Verification items for the finished model (mm, model axes). A direction names the side the tool comes from. Give positions to 0.01 mm unless a question says otherwise; leave off trailing zeros. Order: outer loops, then holes, each group sorted by start corner. A loop starts at its lowest first (then second) coordinate and runs counter-clockwise, first axis right, second up.
(1) Mould release check, pull along Z, two halves, no side actions. Record for faces 5 (the face through (-43, 2, -21.897)), 6 (the face through (-26.148, 1.933, -20.883)), 7 (the face through (-42, 3, -12)): pulls with the +Z half, pulls with the -Z half, needs draft (parallel to the pull), parting line crosses it, or undercut.
(2) Sectioned sample at A-A on z = -11.5. Record the cut outline in (x, y).
(3) Sectioned sample at B-B on x = -23. Record the cut outline in (y, z).
(4) Access from +Z, -Z, +X, -X, +Y, -Y to the whole of each face (thin tool, end or side, straight path). Record for faces 1 (the face through (-8.947, 2, -12)), 2 (the face through (-44.06, 2.23, -20.88)), 3 (the face through (-21.675, 2, -11)), 4 (the face through (-30, 2, -18.897)).
(5) Gauge pin test, flat ends, axial feed: pin 1 (2.5 mm diameter, centred on x = -25, y = 3, fed in from +Z); pin 2 (1.2 mm diameter, centred on x = -44, y = 2.5, fed in from +Z); pin 3 (0.8 mm diameter, centred on y = 1.5, z = -19.5, fed in from -X). Record the tip position at first contact, or that the pin passes through.
(6) Scan lines: L1, parallel to X at y = 2.5, z = -19; L2, parallel to X at y = 1.75, z = 0; L3, parallel to X at y = 2, z = -13. Record each from-to range of solid material in increasing order.
```python
from build123d import *

# Parameters (mm, degrees)
SKETCH1_W            = 55
SKETCH1_H            = 30
BOSS_EXTRUDE1_DEPTH  = 1
SKETCH2_W            = 19.491695939
SKETCH2_H            = 7.592367472
BOSS_EXTRUDE2_DEPTH  = 1
SKETCH3_W            = 17.868683869
SKETCH3_H            = 5.806480893
BOSS_EXTRUDE3_DEPTH  = 5
SKETCH4_R            = 1.387992379
SKETCH4_R_2          = 1.271029941
SKETCH4_R_3          = 1.252160081
SKETCH4_R_4          = 1.29898612
SKETCH4_R_5          = 1.250669325
CUT_EXTRUDE1_DEPTH   = 1
SKETCH5_W            = 10.590314041
SKETCH5_H            = 7.273255242
BOSS_EXTRUDE4_DEPTH  = 1
SKETCH6_W            = 9.57185552
SKETCH6_H            = 5.896073661
BOSS_EXTRUDE5_DEPTH  = 5
SKETCH7_R            = 1.704864166
SKETCH7_R_2          = 1.652773159
CUT_EXTRUDE2_DEPTH   = 1
SKETCH8_W            = 4.39691748
SKETCH8_H            = 1.56078367
SKETCH8_H_2          = 1.965861173
SKETCH8_H_3          = 1.923435972
BOSS_EXTRUDE6_DEPTH  = 3
SKETCH9_W            = 3.511257789
SKETCH9_H            = 7.74384092
SKETCH9_W_2          = 2.828211164
SKETCH9_W_3          = 3.357629357
SKETCH9_H_2          = 9.12002374
SKETCH9_W_4          = 3.515822041
BOSS_EXTRUDE7_DEPTH  = 2
SKETCH11_W           = 9.526847307
SKETCH11_H           = 2.580834009
BOSS_EXTRUDE9_DEPTH  = 1
SKETCH12_W           = 10.214883885
SKETCH12_H           = 2.399198827
BOSS_EXTRUDE10_DEPTH = 1
SKETCH13_W           = 9.211002793
SKETCH13_H           = 2.314821269
BOSS_EXTRUDE11_DEPTH = 1
SKETCH14_W           = 8.269131958
SKETCH14_H           = 2.253083688
BOSS_EXTRUDE12_DEPTH = 1
SKETCH15_R           = 2.31957405
SKETCH15_R_2         = 2.335420551
SKETCH15_R_3         = 2.850653073
SKETCH15_R_4         = 3.324876744
BOSS_EXTRUDE13_DEPTH = 5
SKETCH16_R           = 1.17518149
SKETCH16_R_2         = 1.252285298
SKETCH16_R_3         = 1.321478457
SKETCH16_R_4         = 1.276209415
CUT_EXTRUDE3_DEPTH   = 5
SKETCH17_W           = 3.572088618
SKETCH17_H           = 5.777043793
SKETCH17_W_2         = 3.071926892
SKETCH17_H_2         = 6.434501435
CUT_EXTRUDE4_DEPTH   = 5
SKETCH18_W           = 6.981016606
SKETCH18_H           = 6.578879703
SKETCH18_W_2         = 3.086522126
SKETCH18_H_2         = 3.227214814
SKETCH18_W_3         = 3.221722133
SKETCH18_H_3         = 3.240258565
SKETCH18_W_4         = 3.482439067
SKETCH18_H_4         = 3.404908775
BOSS_EXTRUDE14_DEPTH = 2
SKETCH19_R           = 0.719775063
SKETCH19_R_2         = 0.76029107
SKETCH19_R_3         = 0.758288133
SKETCH19_R_4         = 0.716718546
SKETCH19_R_5         = 0.645890237
SKETCH19_R_6         = 0.78925264
SKETCH19_R_7         = 0.788868737
SKETCH19_R_8         = 0.878549595
SKETCH19_R_9         = 0.90829019
SKETCH19_R_10        = 0.920218082
SKETCH19_R_11        = 0.847809832
SKETCH19_R_12        = 0.813287674
BOSS_EXTRUDE15_DEPTH = 2
SKETCH20_W           = 2.420557599
SKETCH20_H           = 3.478717889
BOSS_EXTRUDE17_DEPTH = 4
SKETCH22_W           = 1.956579844
SKETCH22_H           = 2.647802663
BOSS_EXTRUDE19_DEPTH = 4
SKETCH23_R           = 0.740483371
BOSS_EXTRUDE20_DEPTH = 3


with BuildPart() as part:
    # Sketch1 → Boss-Extrude1 (new body)
    with BuildSketch(Plane(origin=(0, 0, 0), x_dir=(1, 0, 0), z_dir=(0, 1, 0))):
        with Locations((-21.264064322, 3.89729895)):
            Rectangle(SKETCH1_W, SKETCH1_H)
    extrude(amount=BOSS_EXTRUDE1_DEPTH)

    # Sketch2 → Boss-Extrude2 (add)
    with BuildSketch(Plane(origin=(0, 1, 0), x_dir=(1, 0, 0), z_dir=(0, 1, 0))):
        with Locations((-5.49817758, -4.994329297)):
            Rectangle(SKETCH2_W, SKETCH2_H)
    extrude(amount=BOSS_EXTRUDE2_DEPTH)

    # Sketch3 → Boss-Extrude3 (add)
    with BuildSketch(Plane(origin=(0, 2, 0), x_dir=(1, 0, 0), z_dir=(0, 1, 0))):
        with Locations((-5.399712824, -5.130077774)):
            Rectangle(SKETCH3_W, SKETCH3_H)
    extrude(amount=BOSS_EXTRUDE3_DEPTH)

    # Sketch4 → Cut-Extrude1 (cut)
    with BuildSketch(Plane(origin=(0, 7, 0), x_dir=(1, 0, 0), z_dir=(0, 1, 0))):
        with Locations(Location((-12.18713871, -5.16756273, 0), (0, 0, 270))):
            Circle(SKETCH4_R)
        with Locations(Location((-8.689373295, -5.16756273, 0), (0, 0, 270))):
            Circle(SKETCH4_R_2)
        with Locations(Location((-5.533968846, -5.16756273, 0), (0, 0, 270))):
            Circle(SKETCH4_R_3)
        with Locations(Location((-2.349125846, -5.16756273, 0), (0, 0, 270))):
            Circle(SKETCH4_R_4)
        with Locations(Location((0.92403281, -5.16756273, 0), (0, 0, 270))):
            Circle(SKETCH4_R_5)
    extrude(amount=-CUT_EXTRUDE1_DEPTH, mode=Mode.SUBTRACT)

    # Sketch5 → Boss-Extrude4 (add)
    with BuildSketch(Plane(origin=(0, 1, 0), x_dir=(1, 0, 0), z_dir=(0, 1, 0))):
        with Locations((-20.994245653, -4.916719061)):
            Rectangle(SKETCH5_W, SKETCH5_H)
    extrude(amount=BOSS_EXTRUDE4_DEPTH)

    # Sketch6 → Boss-Extrude5 (add)
    with BuildSketch(Plane(origin=(0, 2, 0), x_dir=(1, 0, 0), z_dir=(0, 1, 0))):
        with Locations((-21.014512422, -4.903762727)):
            Rectangle(SKETCH6_W, SKETCH6_H)
    extrude(amount=BOSS_EXTRUDE5_DEPTH)

    # Sketch7 → Cut-Extrude2 (cut)
    with BuildSketch(Plane(origin=(0, 7, 0), x_dir=(1, 0, 0), z_dir=(0, 1, 0))):
        with Locations(Location((-23.578627502, -4.834787204, 0), (0, 0, 270))):
            Circle(SKETCH7_R)
        with Locations(Location((-19.287367013, -4.834787204, 0), (0, 0, 270))):
            Circle(SKETCH7_R_2)
    extrude(amount=-CUT_EXTRUDE2_DEPTH, mode=Mode.SUBTRACT)

    # Sketch8 → Boss-Extrude6 (add)
    with BuildSketch(Plane(origin=(0, 1, 0), x_dir=(1, 0, 0), z_dir=(0, 1, 0))):
        with Locations((-23.873740649, 14.984908312)):
            Rectangle(SKETCH8_W, SKETCH8_H)
        with Locations((-23.873740649, 11.393249572)):
            Rectangle(SKETCH8_W, SKETCH8_H_2)
        with Locations((-23.873740649, 7.106266144)):
            Rectangle(SKETCH8_W, SKETCH8_H_3)
    extrude(amount=BOSS_EXTRUDE6_DEPTH)

    # Sketch9 → Boss-Extrude7 (add)
    with BuildSketch(Plane(origin=(0, 1, 0), x_dir=(1, 0, 0), z_dir=(0, 1, 0))):
        with Locations((-41.824470852, 11.59406106)):
            Rectangle(SKETCH9_W, SKETCH9_H)
        with Locations((-34.376000541, 11.59406106)):
            Rectangle(SKETCH9_W_2, SKETCH9_H)
        with Locations((-10.62597461, 12.28215247)):
            Rectangle(SKETCH9_W_3, SKETCH9_H_2)
        with Locations((-4.140862927, 12.28215247)):
            Rectangle(SKETCH9_W_4, SKETCH9_H_2)
    extrude(amount=BOSS_EXTRUDE7_DEPTH)

    # Sketch11 → Boss-Extrude9 (add)
    with BuildSketch(Plane(origin=(0, 0, -18.89729895), x_dir=(-1, 0, 0), z_dir=(0, 0, -1))):
        with Locations((43.030759371, 2.129646377)):
            Rectangle(SKETCH11_W, SKETCH11_H)
    extrude(amount=BOSS_EXTRUDE9_DEPTH)

    # Sketch12 → Boss-Extrude10 (add)
    with BuildSketch(Plane(origin=(0, 0, -18.89729895), x_dir=(-1, 0, 0), z_dir=(0, 0, -1))):
        with Locations((30.43046596, 2.006084235)):
            Rectangle(SKETCH12_W, SKETCH12_H)
    extrude(amount=BOSS_EXTRUDE10_DEPTH)

    # Sketch13 → Boss-Extrude11 (add)
    with BuildSketch(Plane(origin=(0, 0, -18.89729895), x_dir=(-1, 0, 0), z_dir=(0, 0, -1))):
        with Locations((12.330175076, 2.015979145)):
            Rectangle(SKETCH13_W, SKETCH13_H)
    extrude(amount=BOSS_EXTRUDE11_DEPTH)

    # Sketch14 → Boss-Extrude12 (add)
    with BuildSketch(Plane(origin=(0, 0, -18.89729895), x_dir=(-1, 0, 0), z_dir=(0, 0, -1))):
        with Locations((1.581311109, 1.994768123)):
            Rectangle(SKETCH14_W, SKETCH14_H)
    extrude(amount=BOSS_EXTRUDE12_DEPTH)

    # Sketch15 → Boss-Extrude13 (add)
    with BuildSketch(Plane(origin=(0, 1, 0), x_dir=(1, 0, 0), z_dir=(0, 1, 0))):
        with Locations(Location((-7.252523926, 2.900653957, 0), (0, 0, 270))):
            Circle(SKETCH15_R)
        with Locations(Location((-1.058148133, 2.900653957, 0), (0, 0, 270))):
            Circle(SKETCH15_R_2)
        with Locations(Location((-33.782017374, -5.710655696, 0), (0, 0, 270))):
            Circle(SKETCH15_R_3)
        with Locations(Location((-43.660307349, -5.710655696, 0), (0, 0, 270))):
            Circle(SKETCH15_R_4)
    extrude(amount=BOSS_EXTRUDE13_DEPTH)

    # Sketch16 → Cut-Extrude3 (cut)
    with BuildSketch(Plane(origin=(0, 1, 0), x_dir=(1, 0, 0), z_dir=(0, 1, 0))):
        with Locations((-51.576522497, 22.016727671)):
            Circle(SKETCH16_R)
        with Locations((-51.576522497, -8.848199257)):
            Circle(SKETCH16_R_2)
        with Locations((4.236348916, 22.016727671)):
            Circle(SKETCH16_R_3)
        with Locations(Location((4.71641652, -9.248882224, 0), (0, 0, 270))):
            Circle(SKETCH16_R_4)
    extrude(amount=-CUT_EXTRUDE3_DEPTH, mode=Mode.SUBTRACT)

    # Sketch17 → Cut-Extrude4 (cut)
    with BuildSketch(Plane(origin=(0, 1, 0), x_dir=(1, 0, 0), z_dir=(0, 1, 0))):
        with Locations((-52.185475992, 15.830959354)):
            Rectangle(SKETCH17_W, SKETCH17_H)
        with Locations((5.809579957, 14.174599881)):
            Rectangle(SKETCH17_W_2, SKETCH17_H_2)
    extrude(amount=-CUT_EXTRUDE4_DEPTH, mode=Mode.SUBTRACT)

    # Sketch18 → Boss-Extrude14 (add)
    with BuildSketch(Plane(origin=(0, 1, 0), x_dir=(1, 0, 0), z_dir=(0, 1, 0))):
        with Locations((-33.773534226, 1.886893529)):
            Rectangle(SKETCH18_W, SKETCH18_H)
        with Locations((-46.681665239, 4.480707082)):
            Rectangle(SKETCH18_W_2, SKETCH18_H_2)
        with Locations((-41.483525563, 0.631278088)):
            Rectangle(SKETCH18_W_3, SKETCH18_H_3)
        with Locations((-17.396903315, 16.139817099)):
            Rectangle(SKETCH18_W_4, SKETCH18_H_4)
    extrude(amount=BOSS_EXTRUDE14_DEPTH)

    # Sketch19 → Boss-Extrude15 (add)
    with BuildSketch(Plane(origin=(0, 0, -19.89729895), x_dir=(-1, 0, 0), z_dir=(0, 0, -1))):
        with Locations((-1.366958386, 1.973684487)):
            Circle(SKETCH19_R)
        with Locations((1.106822062, 1.973684487)):
            Circle(SKETCH19_R_2)
        with Locations((3.600495928, 1.795519179)):
            Circle(SKETCH19_R_3)
        with Locations((9.279826449, 1.973684487)):
            Circle(SKETCH19_R_4)
        with Locations((11.619345424, 1.795519179)):
            Circle(SKETCH19_R_5)
        with Locations((14.413821044, 1.795519179)):
            Circle(SKETCH19_R_6)
        with Locations((26.935713498, 1.898398295)):
            Circle(SKETCH19_R_7)
        with Locations((29.585968295, 1.898398295)):
            Circle(SKETCH19_R_8)
        with Locations((32.353085369, 1.898398295)):
            Circle(SKETCH19_R_9)
        with Locations((40.159649939, 1.898398295)):
            Circle(SKETCH19_R_10)
        with Locations((43.252965878, 1.973684487)):
            Circle(SKETCH19_R_11)
        with Locations((45.626690014, 1.973684487)):
            Circle(SKETCH19_R_12)
    extrude(amount=BOSS_EXTRUDE15_DEPTH)

    # Sketch20 → Boss-Extrude17 (add)
    with BuildSketch(Plane(origin=(0, 1, 0), x_dir=(1, 0, 0), z_dir=(0, 1, 0))):
        with Locations((-45.209433873, -0.39597322)):
            Rectangle(SKETCH20_W, SKETCH20_H)
    extrude(amount=BOSS_EXTRUDE17_DEPTH)

    # Sketch22 → Boss-Extrude19 (add)
    with BuildSketch(Plane(origin=(0, 1, 0), x_dir=(1, 0, 0), z_dir=(0, 1, 0))):
        with Locations((3.480988959, 4.090806431)):
            Rectangle(SKETCH22_W, SKETCH22_H)
    extrude(amount=BOSS_EXTRUDE19_DEPTH)

    # Sketch23 → Boss-Extrude20 (add)
    with BuildSketch(Plane(origin=(4.459278881, 0, 0), x_dir=(0, 0, -1), z_dir=(1, 0, 0))):
        with Locations(Location((4.071876489, 3.501691713, 0), (0, 0, 180))):
            Circle(SKETCH23_R)
    extrude(amount=BOSS_EXTRUDE20_DEPTH)


solid = part.part
```
Ans:
1. face 5: pulls with the -Z half
1. face 6: needs draft
1. face 7: undercut
2. outline: (-48.76, 0) - (4.27, 0) - (4.27, 1) - (-2.38, 1) - (-2.38, 3) - (-5.9, 3) - (-5.9, 1) - (-8.95, 1) - (-8.95, 3) - (-12.3, 3) - (-12.3, 1) - (-21.68, 1) - (-21.68, 4) - (-26.07, 4) - (-26.07, 1) - (-32.96, 1) - (-32.96, 3) - (-35.79, 3) - (-35.79, 1) - (-40.07, 1) - (-40.07, 3) - (-43.58, 3) - (-43.58, 1) - (-48.76, 1) - close
3. outline: (0, -18.9) - (1, -18.9) - (1, -15.77) - (4, -15.77) - (4, -14.2) - (1, -14.2) - (1, -12.38) - (4, -12.38) - (4, -10.41) - (1, -10.41) - (1, -8.07) - (4, -8.07) - (4, -6.14) - (1, -6.14) - (1, 1.28) - (2, 1.28) - (2, 1.96) - (7, 1.96) - (7, 3.23) - (6, 3.23) - (6, 6.44) - (7, 6.44) - (7, 7.85) - (2, 7.85) - (2, 8.55) - (1, 8.55) - (1, 11.1) - (0, 11.1) - close
4. face 1: +Y
4. face 2: -Z
4. face 3: -Z, +Y
4. face 4: +X, -X, +Y
5. pin 1: stops at z = 8.55
5. pin 2: stops at z = 9.04
5. pin 3: stops at x = -47.79
6. L1: x = -47.79 to -38.27, -35.54 to -25.32, -16.94 to -7.72, -5.72 to 2.55
6. L2: x = -46.42 to -44, -43.09 to -39.87, -37.26 to -30.28
6. L3: x = -43.58 to -40.07, -35.79 to -32.96, -12.3 to -8.95, -5.9 to -2.38
